from build123d import *

# Parameters (mm, degrees)
BOSS_EXTRUDE1_DEPTH = 50.8
SKETCH3_W           = 25.4
SKETCH3_H           = 25.4
CUT_EXTRUDE1_DEPTH  = 25.4
SKETCH8_W           = 24.892
SKETCH8_H           = 24.892
BOSS_EXTRUDE2_DEPTH = 24.892
SKETCH12_R          = 3.429
CUT_EXTRUDE2_DEPTH  = 25.4
SKETCH13_W          = 25.4
SKETCH13_H          = 12.7
CUT_EXTRUDE3_DEPTH  = 25.908
FILLET1_R           = 2.54
SKETCH14_R          = 3.175
CUT_EXTRUDE5_DEPTH  = 246.663470197
CUT_EXTRUDE6_DEPTH  = 5.08


with BuildPart() as part:
    # Sketch2 → Boss-Extrude1 (new body)
    with BuildSketch(Plane(origin=(0, 0, 0), x_dir=(1, 0, 0), z_dir=(0, 1, 0))):
        Polygon((-50.8, 155.575), (0, 155.575), (0, 0), (107.95, 0), (107.95, -50.8), (-50.8, -50.8), align=None)
    extrude(amount=BOSS_EXTRUDE1_DEPTH)

    # Sketch3 → Cut-Extrude1 (cut)
    with BuildSketch(Plane(origin=(107.95, 0, 0), x_dir=(0, 0, -1), z_dir=(1, 0, 0))):
        with Locations((-25.239912, 25.560088)):
            Rectangle(SKETCH3_W, SKETCH3_H)
    extrude(amount=-CUT_EXTRUDE1_DEPTH, mode=Mode.SUBTRACT)

    # Sketch7 → CBORE for 1/4 Binding Head Machine Screw1 (revolve, cut)
    with BuildSketch(Plane(origin=(95.25, 50.8, 25.4), x_dir=(0, 0, 1), z_dir=(1, 0, 0))):
        Polygon((0, 0), (0, 50.8), (3.3782, 50.8), (3.3782, 4.191), (7.14375, 4.191), (7.14375, 0.635), (7.77875, 0), align=None)
    revolve(axis=Axis((95.25, 57.15, 25.4), (0, -1, 0)), mode=Mode.SUBTRACT)

    # Sketch8 → Boss-Extrude2 (add)
    with BuildSketch(Plane(origin=(0, 0, -155.575), x_dir=(-1, 0, 0), z_dir=(0, 0, -1))):
        with Locations((25.4, 25.4)):
            Rectangle(SKETCH8_W, SKETCH8_H)
    extrude(amount=BOSS_EXTRUDE2_DEPTH)

    # Sketch12 → Cut-Extrude2 (cut)
    with BuildSketch(Plane(origin=(0, 37.846, 0), x_dir=(1, 0, 0), z_dir=(0, 1, 0))):
        with Locations(Location((-25.4, 168.275, 0), (0, 0, 270))):
            Circle(SKETCH12_R)
    extrude(amount=-CUT_EXTRUDE2_DEPTH, mode=Mode.SUBTRACT)

    # Sketch13 → Cut-Extrude3 (cut)
    with BuildSketch(Plane(origin=(0, 50.8, 0), x_dir=(1, 0, 0), z_dir=(0, 1, 0))):
        with Locations((-25.4, 117.475)):
            Rectangle(SKETCH13_W, SKETCH13_H)
    extrude(amount=-CUT_EXTRUDE3_DEPTH, mode=Mode.SUBTRACT)

    # Fillet1
    fillet1_edges = [part.edges().sort_by_distance(p)[0] for p in [
        (-38.1, 50.8, -117.475),
        (-12.7, 50.8, -117.475),
    ]]
    fillet(fillet1_edges, radius=FILLET1_R)

    # Sketch14 → Cut-Extrude5 (cut, through all)
    with BuildSketch(Plane.ZY.offset(50.8)):
        with Locations((-117.475, 38.1)):
            Circle(SKETCH14_R)
    extrude(amount=-CUT_EXTRUDE5_DEPTH, mode=Mode.SUBTRACT)

    # Sketch17 → Cut-Extrude6 (cut)
    with BuildSketch(Plane(origin=(0, 50.8, 0), x_dir=(1, 0, 0), z_dir=(0, 1, 0))):
        Polygon((0, 155.575), (0, 0), (107.95, 0), (107.95, -7.62), (-7.62, -7.62), (-7.62, 155.575), align=None)
    extrude(amount=-CUT_EXTRUDE6_DEPTH, mode=Mode.SUBTRACT)


solid = part.part
The model under review builds one solid part; all positions refer to its coordinate system, in mm. A direction names the side the tool comes from. Coordinates: 2 decimals unless noted, no trailing zeros. Write each loop counter-clockwise with the first axis right and the second up, starting at its lowest first coordinate (ties: lowest second). Pieces come first, ordered by that corner, then holes. Notation, with made-up numbers: M 83,33 L 117,33 A10 cw 117,49 Z; hole C 45.25,47 d6. An arc over 180 degrees is marked long. Put each result on its own line as item: value.
1) Draft analysis for pull direction Y (two halves, no side actions). For faces 1 (the flat face through (95, 25, 37.94)), 2 (the flat face through (30, 25, 50.8)), 3 (the flat face through (97, 46.609, 22)), 4 (the flat face through (-28, 12.954, -171)), state which applies: released by +Y, released by -Y, zero draft, split by the parting line, or undercut.
Computed:
face 1: undercut
face 2: zero draft
face 3: released by +Y
face 4: released by -Y
2) Add section A-A on x = -25.4. Give the boundary of the cut face in (y, z) (3 decimals), then the cut area to 3 significant figures.
Computed:
outline: M 0,-155.575 L 12.954,-155.575 L 12.954,-164.846 L 37.846,-164.846 L 37.846,-155.575 L 50.8,-155.575 L 50.8,-123.825 L 24.892,-123.825 L 24.892,-111.125 L 50.8,-111.125 L 50.8,50.8 L 0,50.8 Z; M 12.954,-180.467 L 37.846,-180.467 L 37.846,-171.704 L 12.954,-171.704 Z
area: 10,600 mm2
3) For faces 5 (the flat face through (0, 23, -79)), 6 (the flat face through (-38.1, 34, -117)), 7 (the flat face through (-28, 37.846, -171)), 8 (the flat face through (82.55, 26, 25)), list the 3-axis set-ups (+Z, -Z, +X, -X, +Y, -Y) from which the entire face can be reached by the end or side of a thin tool; tool diameter is ignored.
Computed:
face 5: -Z, +X, +Y, -Y
face 6: +Y
face 7: -Z, +X, -X, +Y
face 8: +X
4) Add section C-C on y = 28. Give the boundary of the cut face in (x, z) (3 decimals), then the cut area to 3 significant figures.
Computed:
outline: M -50.8,-155.575 L -37.846,-155.575 L -37.846,-180.467 L -12.954,-180.467 L -12.954,-155.575 L 0,-155.575 L 0,0 L 107.95,0 L 107.95,12.54 L 82.55,12.54 L 82.55,37.94 L 107.95,37.94 L 107.95,50.8 L -50.8,50.8 Z; hole M -38.1,-123.825 L -12.7,-123.825 L -12.7,-111.125 L -38.1,-111.125 Z; hole C -25.4,-168.275 d6.858
area: 15,600 mm2
5) Add section B-B on y = 8. Give the boundary of the cut face in (x, z) (3 decimals).
Computed:
outline: M -50.8,-155.575 L 0,-155.575 L 0,0 L 107.95,0 L 107.95,50.8 L -50.8,50.8 Z; hole C 95.25,25.4 d6.756
6) Add section D-D on z = 25.4. Give the boundary of the cut face in (x, y) (3 decimals).
Computed:
outline: M -50.8,0 L 91.872,0 L 91.872,12.86 L 82.55,12.86 L 82.55,38.26 L 91.872,38.26 L 91.872,46.609 L 88.106,46.609 L 88.106,50.165 L 87.471,50.8 L -50.8,50.8 Z; M 98.628,0 L 107.95,0 L 107.95,12.86 L 98.628,12.86 Z; M 98.628,38.26 L 107.95,38.26 L 107.95,50.8 L 103.029,50.8 L 102.394,50.165 L 102.394,46.609 L 98.628,46.609 Z
7) Wall thickness on probe 1 along Z at (x, y) = (-24, 42) (3 decimals); probe 2 along Z at (x, y) = (95.25, 48.7); probe 3 along Z at (x, y) = (-25, 28) (3 decimals): over which ranges is each line inside the solid? List them lowest first. Write a range as [from, to].
Computed:
probe 1: z = [-155.575, -123.825], [-111.125, 50.8]
probe 2: z = [7.62, 18.26], [32.54, 50.8]
probe 3: z = [-180.467, -171.681], [-164.869, -123.825], [-111.125, 50.8]
8) Clearance check with flat-ended pins moving along their axes: pin 1 Ø12.5 at (y, z) = (31, -171.5) entering from -X; pin 2 Ø7.5 at (x, y) = (98, 30) entering from -Z; pin 3 Ø2.5 at (y, z) = (49.5, -42) entering from +X; pin 4 Ø4 at (x, z) = (95.25, 25.4) entering from +Y. State where each tip first meets the part, or that it passes through.
Computed:
pin 1: stops at x = -37.85
pin 2: stops at z = 0
pin 3: stops at x = -7.62
pin 4: passes through
